from build123d import *

# Parameters (mm, degrees)
F1_DEPTH = 15


with BuildPart() as f1:
    # F0 (on Front) → F1 (new body)
    with BuildSketch(Plane.XZ):
        with BuildLine():
            ThreePointArc((25.24413, 26.290931), (14.382766, 16.172523), (0, 12.5))
            ThreePointArc((0, 12.5), (-11.921462, 3.758822), (-7.169705, -10.239401))
            Line((-7.169705, -10.239401), (0, -15.259682))
            Line((0, -15.259682), (7.169705, -10.239401))
            ThreePointArc((7.169705, -10.239401), (7.730124, -10.115159), (8.214252, -10.423582))
            Line((8.214252, -10.423582), (11.082134, -14.519342))
            Line((11.082134, -14.519342), (11.49171, -14.232554))
            Line((11.49171, -14.232554), (8.623828, -10.136794))
            ThreePointArc((8.623828, -10.136794), (7.816948, -9.622755), (6.882917, -9.829825))
            Line((6.882917, -9.829825), (0, -14.649295))
            Line((0, -14.649295), (-6.882917, -9.829825))
            ThreePointArc((-6.882917, -9.829825), (-11.444604, 3.60847), (0, 12))
            ThreePointArc((0, 12), (14.622479, 15.733732), (25.664865, 26.02078))
            Line((25.664865, 26.02078), (25.24413, 26.290931))
        make_face()
        with BuildLine():
            ThreePointArc((-7.169705, -10.239401), (-11.921462, 3.758822), (0, 12.5))
            ThreePointArc((0, 12.5), (14.382766, 16.172523), (25.24413, 26.290931))
            Line((25.24413, 26.290931), (24.823395, 26.561081))
            ThreePointArc((24.823395, 26.561081), (14.143054, 16.611314), (0, 12.999999))
            ThreePointArc((0, 12.999999), (-12.39832, 3.909175), (-7.456493, -10.648976))
            Line((-7.456493, -10.648976), (0, -15.870069))
            Line((0, -15.870069), (7.456493, -10.648976))
            ThreePointArc((7.456493, -10.648976), (7.6433, -10.607562), (7.804677, -10.71037))
            Line((7.804677, -10.71037), (10.672559, -14.80613))
            Line((10.672559, -14.80613), (11.082134, -14.519342))
            Line((11.082134, -14.519342), (8.214252, -10.423582))
            ThreePointArc((8.214252, -10.423582), (7.730124, -10.115159), (7.169705, -10.239401))
            Line((7.169705, -10.239401), (0, -15.259682))
            Line((0, -15.259682), (-7.169705, -10.239401))
        make_face()
    extrude(amount=F1_DEPTH)


solid = f1.part
Geometry: final body of the model. Coordinates: model frame, mm. A direction names the side the tool comes from. Give positions to 0.01 mm unless a question says otherwise; leave off trailing zeros. Write each loop counter-clockwise with the first axis right and the second up, starting at its lowest first coordinate (ties: lowest second). Pieces come first, ordered by that corner, then holes.
(1) Ray query, line 1 (X direction, y = -5.25, z = -12); line 2 (Z direction, x = -8.5, y = -7.75); line 3 (Z direction, x = -3, y = -10). Return the intervals inside material, ascending.
(2) Cut plane D-D, the plane z = 18. Return loops of the section in (x, y).
(3) Mould query, pull axis Z, two halves, no side actions, for faces 1 (the flat face through (-3.393, -7.395, -12.273)), 2 (the flat face through (-4, 0, 12)), 3 (the cylindrical face through (-12.327, -7.395, 4.128)), 4 (the flat face through (9.2, -7.4, -12.7)). Classes: released by +Z, released by -Z, zero draft, split by the parting line, or undercut.
(4) Cut plane C-C, the plane x = 2.5. Return loops of the section in (y, z), then the cut area to 3 significant figures.
(5) Cut plane B-B, the plane y = -12.25. Return loops of the section in (x, z), then the cut area to 3 significant figures.
(6) First-contact query: P1, Ø4, axis at y = -8.5, z = 3, coming from the +X side; P2, Ø1.5, axis at x = -5.5, y = -12.5, coming from the -Z side; P3, Ø1.5, axis at x = -5.5, y = -2.5, coming from the +Z side. Flat tips, straight axial feed; report the tip coordinate or a pass-through.
(7) Access query for faces 5 (the flat face through (-4, -15, 12)), 6 (the flat face through (3.676, -7.395, -13.296)), 7 (the flat face through (10.078, -7.395, -12.213)), 8 (the cylindrical face through (14.32, -7.4, 16.71)), 9 (the cylindrical face through (7.83, -7.395, -9.625)). Directions: +Z, -Z, +X, -X, +Y, -Y. A direction counts if a zero-diameter tool reaches every point of the face in a straight line with its end or side. Return the directions, or none.
(8) Cut plane A-A, the plane x = -8. Return loops of the section in (y, z).
Values follow:
1. line 1: x = -5.53 to -3.78, 3.78 to 5.53, 8.71 to 9.93
1. line 2: z = -9.84 to -8.47, 8.47 to 9.84
1. line 3: z = -13.77 to -12.55, 11.62 to 12.65
2. outline: (16.43, -15) - (18.17, -15) - (18.17, 0) - (16.43, 0) - close
3. face 1: undercut
3. face 2: zero draft
3. face 3: split by the parting line
3. face 4: released by -Z
4. outline: (-15, -14.12) - (0, -14.12) - (0, -12.9) - (-15, -12.9) - close; (-15, 12.1) - (0, 12.1) - (0, 13.11) - (-15, 13.11) - close
4. area: 33.4 mm2
5. outline: (-7.46, -10.65) - (0, -15.87) - (7.46, -10.65) arc R0.25 cw to (7.8, -10.71) - (10.67, -14.81) - (11.08, -14.52) - (11.49, -14.23) - (8.62, -10.14) arc R1.25 ccw to (6.88, -9.83) - (0, -14.65) - (-6.88, -9.83) arc R12 cw to (0, 12) arc R30.5 ccw to (25.66, 26.02) - (25.24, 26.29) - (24.82, 26.56) arc R29.5 cw to (0, 13) arc R13 ccw to start
5. area: 85.3 mm2
6. P1: stops at x = -10.91
6. P2: stops at z = -12.54
6. P3: stops at z = 12.1
7. face 5: +Z, -Z, +X, -X, -Y
7. face 6: -Z, +Y, -Y
7. face 7: +X, +Y, -Y
7. face 8: +Z, -X, +Y, -Y
7. face 9: +Y, -Y
8. outline: (-15, -10.25) - (0, -10.25) - (0, -8.94) - (-15, -8.94) - close; (-15, 8.94) - (0, 8.94) - (0, 10.25) - (-15, 10.25) - close
